from build123d import *

# Parameters (mm, degrees)
SKETCH_1_R      = 7.352953784
SKETCH_1_R_2    = 6.485613762
EXTRUDE_1_DEPTH = 5
SKETCH_2_W      = 14.323977173
SKETCH_2_H      = 11.973415737
EXTRUDE_2_DEPTH = 5


with BuildPart() as part:
    # 草图1 → 凸台-拉伸1 (new body)
    with BuildSketch(Plane.XY):
        with BuildLine():
            Line((0, 14.12037037), (350, 14.12037037))
            ThreePointArc((350, 14.12037037), (364.12037037, 0), (350, -14.12037037))
            Line((350, -14.12037037), (0, -14.12037037))
            ThreePointArc((0, -14.12037037), (-14.12037037, 0), (0, 14.12037037))
        make_face()
        Circle(SKETCH_1_R, mode=Mode.SUBTRACT)
        with Locations((350, 0)):
            Circle(SKETCH_1_R_2, mode=Mode.SUBTRACT)
    extrude(amount=EXTRUDE_1_DEPTH)

    # 草图2 → 凸台-拉伸2 (add)
    with BuildSketch(Plane.XY):
        with Locations((7.161988587, 20.107078239)):
            Rectangle(SKETCH_2_W, SKETCH_2_H)
    extrude(amount=EXTRUDE_2_DEPTH)


solid = part.part
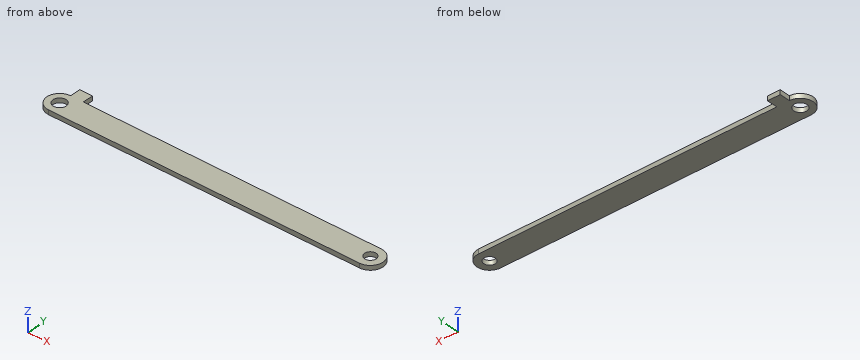
For this review, take the finished solid that the model builds, in its own axes (mm). Give positions to 0.01 mm unless a question says otherwise; leave off trailing zeros. Loops run counter-clockwise (first coordinate to the right, second up) from the corner with the lowest first, then second, coordinate; pieces in that order, holes last.
Item 1: Take a section at B-B, the plane y = 0. State the section outline as (x, z) points.
Item 2: Insertion check: pin 1 (3 mm diameter, centred on y = 9.5, z = 4, fed in from -X); pin 2 (1.5 mm diameter, centred on y = 19.5, z = 3, fed in from -X); pin 3 (2.5 mm diameter, centred on x = 229, z = 2.5, fed in from +Y). Each pin has a flat end and moves straight along its axis. Give the tip position at first contact, or say it passes through.
Item 3: Take a section at A-A, the plane z = 2.2. State the section outline as (x, y) points, and give its area (3 significant figures).
Item 4: For line 1 along Y through (x, z) = (350, 1.15); line 2 along X through (y, z) = (5.5, 2.55); line 3 along X through (y, z) = (-4, 0.3), list the stretches that pass through material, from the lowest coordinate up.
Item 5: Take a section at C-C, the plane x = 295.5. State the section outline as (y, z) points, and give its area (3 significant figures).
Item 6: Take a section at D-D, the plane y = 22. State the section outline as (x, z) points, and give its area (3 significant figures).
Calculated:
1. outline: (-14.12, 0) - (-7.35, 0) - (-7.35, 5) - (-14.12, 5) - close; (7.35, 0) - (343.51, 0) - (343.51, 5) - (7.35, 5) - close; (356.49, 0) - (364.12, 0) - (364.12, 5) - (356.49, 5) - close
2. pin 1: stops at x = -11.64
2. pin 2: stops at x = 0
2. pin 3: stops at y = 14.12
3. outline: (0, -14.12) - (350, -14.12) arc R14.12 ccw to (350, 14.12) - (14.32, 14.12) - (14.32, 26.09) - (0, 26.09) - (0, 14.12) arc R14.12 ccw to start; hole circle Ø14.71 at (0, 0); hole circle Ø12.97 at (350, 0)
3. area: 10,400 mm2
4. line 1: y = -14.12 to -6.49, 6.49 to 14.12
4. line 2: x = -13.01 to -4.88, 4.88 to 346.56, 353.44 to 363.01
4. line 3: x = -13.54 to -6.17, 6.17 to 344.89, 355.11 to 363.54
5. outline: (-14.12, 0) - (14.12, 0) - (14.12, 5) - (-14.12, 5) - close
5. area: 141 mm2
6. outline: (0, 0) - (14.32, 0) - (14.32, 5) - (0, 5) - close
6. area: 71.6 mm2
